Work out the finished part from the listing and answer in its coordinate system (mm). Face numbers are marked on the shaded views. A direction names the side the tool comes from. Coordinates: 2 decimals unless noted, no trailing zeros. Loops run counter-clockwise (first coordinate to the right, second up) from the corner with the lowest first, then second, coordinate; pieces in that order, holes last.
```python
from build123d import *

# Parameters (mm, degrees)
F0_R     = 2
F1_DEPTH = 2
F2_DEPTH = 8
F3_R     = 1


with BuildPart() as f1:
    # F0 (on Top) → F1 (new body)
    with BuildSketch(Plane.XY):
        Polygon((-4, 4.5), (-4, 0), (0, -8), (6.5, -8), (6.5, 4.5), align=None)
        Circle(F0_R, mode=Mode.SUBTRACT)
        Polygon((-4, 6.5), (-4, 4.5), (6.5, 4.5), (6.5, -8), (8.499535, -8.043109), (8.499535, 6.5), align=None)
    extrude(amount=F1_DEPTH)

    # F0 (on Top) → F2 (join)
    with BuildSketch(Plane.XY):
        Polygon((-4, 6.5), (-4, 4.5), (6.5, 4.5), (6.5, -8), (8.499535, -8.043109), (8.499535, 6.5), align=None)
    extrude(amount=F2_DEPTH)

    # F3
    f3_edges = [f1.edges().sort_by_distance(p)[0] for p in [
        (6.5, 4.5, 5),
        (8.499535, 6.5, 4),
        (-4, 6.5, 4),
        (-4, 0, 1),
        (0, -8, 1),
        (8.499535, -8.043109, 4),
    ]]
    fillet(f3_edges, radius=F3_R)


solid = f1.part
```
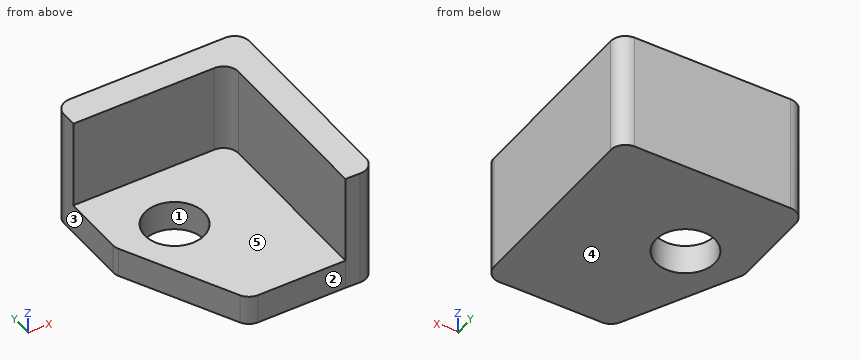
1. A cutting plane is placed at D-D, the plane y = -5.5. Give the vertices of the cut face in (x, z), then the cut area to 3 significant figures.
2. A cutting plane is placed at C-C, the plane z = 4.25. Give the vertices of the cut face in (x, y).
3. A cutting plane is placed at A-A, the plane x = 1.25. Give the vertices of the cut face in (y, z), then the cut area to 3 significant figures.
4. Determine the mould class of the marked faces 1, 2 and 3 for opening direction Y: released by +Y, released by -Y, zero draft, split by the parting line, or undercut.
5. A cutting plane is placed at B-B, the plane y = 0. Give the vertices of the cut face in (x, z).
6. Each of these flat-tipped pins is pushed along its axis until it touches: P1, Ø2, axis at x = 2.5, z = 1, coming from the -Y side; P2, Ø3, axis at x = 1.5, z = 7, coming from the -Y side; P3, Ø5, axis at x = 1.5, y = -0.5, coming from the +Z side. Where does it stop, or does it pass through?
7. For the marked faces 4 and 5, determine the directions among +Z, -Z, +X, -X, +Y, -Y from which every point of the face is accessible in a straight line to the end or side of a thin tool.
8. Straight lines are drawn through the part: probe 1 along Y at (x, z) = (4.5, 6.25); probe 2 along X at (y, z) = (-2.25, 5.5); probe 3 along Z at (x, y) = (5.5, 1). For each, find the intervals that lie inside material, in ascending order.
Answers below:
1. outline: (-1.25, 0) - (8.5, 0) - (8.5, 8) - (6.5, 8) - (6.5, 2) - (-1.25, 2) - close
1. area: 31.5 mm2
2. outline: (-4, 4.5) - (5.5, 4.5) arc R1 cw to (6.5, 3.5) - (6.5, -8) - (7.48, -8.02) arc R1 ccw to (8.5, -7.02) - (8.5, 5.5) arc R1 ccw to (7.5, 6.5) - (-3, 6.5) arc R1 ccw to (-4, 5.5) - close
3. outline: (-8, 0) - (-1.56, 0) - (-1.56, 2) - (-8, 2) - close; (1.56, 0) - (6.5, 0) - (6.5, 8) - (4.5, 8) - (4.5, 2) - (1.56, 2) - close
3. area: 34.8 mm2
4. face 1: undercut
4. face 2: released by -Y
4. face 3: zero draft
5. outline: (-3.97, 0) - (-2, 0) - (-2, 2) - (-3.97, 2) - close; (2, 0) - (8.5, 0) - (8.5, 8) - (6.5, 8) - (6.5, 2) - (2, 2) - close
6. P1: stops at y = -8
6. P2: stops at y = 4.5
6. P3: stops at z = 2
7. face 4: -Z, +X, -X, +Y, -Y
7. face 5: +Z, -X, -Y
8. probe 1: y = 4.5 to 6.5
8. probe 2: x = 6.5 to 8.5
8. probe 3: z = 0 to 2
